Could you check a few things on this drawing? It's one solid part, dimensions in mm from its lowest x, y, z. Give positions to 0.01 mm unless a question says otherwise; leave off trailing zeros. Write each loop counter-clockwise with the first axis right and the second up, starting at its lowest first coordinate (ties: lowest second). Pieces come first, ordered by that corner, then holes. Notation, with made-up numbers: M 84,65 L 102,65 A35 cw 102,97 Z; hole C -32,29.25 d7. An arc over 180 degrees is marked long. Answer as CSV lines item,"result". Start each with the question number.
Q1. If I drill on line 1 along X through (y, z) = (1.5, 140.5) (1 decimal); line 2 along Z through (x, y) = (107.5, 1.5), over which ranges is the centre line in solid material (lowest first)?
Q2. Suppose I cut it at B-B (z = 55.5). Write out the boundary of the cut face in (x, y) (1 decimal).
Q3. For pin 1 (2 mm diameter, centred on y = 4, z = 159.5, fed in from +X); pin 2 (2 mm diameter, centred on y = 5, z = 159.5, fed in from -X); pin 3 (2 mm diameter, centred on x = 176, y = 3.5, fed in from -Z), each with a flat end and sliding along its axis, tell me the tip position at first contact or that it passes through.
Q4. Suppose I cut it at A-A (x = 28.5). Write out the boundary of the cut face in (y, z).
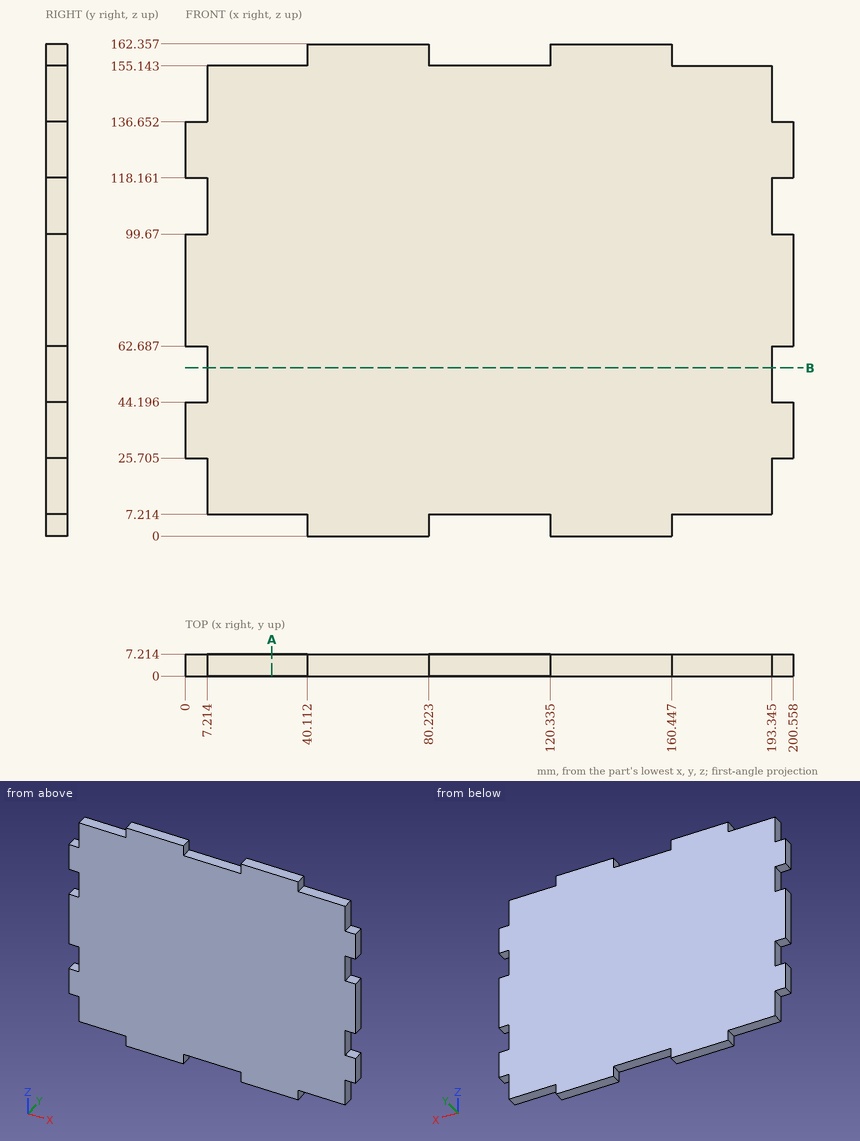
Resolved:
1,line 1,"7.2 to 193.3"
1,line 2,"7.21 to 155.14"
2,outline,"M 7.2,0 L 193.3,0 L 193.3,7.2 L 7.2,7.2 Z"
3,pin 1,"x = 160.45"
3,pin 2,"x = 40.11"
3,pin 3,"z = 7.21"
4,outline,"M 0,7.21 L 7.21,7.21 L 7.21,155.14 L 0,155.14 Z"
